from build123d import *

# Parameters (mm, degrees)
SKETCH1_W           = 16.5
SKETCH1_H           = 16.5
BOSS_EXTRUDE2_DEPTH = 7.5
SKETCH2_W           = 16.5
SKETCH2_H           = 10.25
CUT_EXTRUDE1_DEPTH  = 33.450924486
SKETCH5_W           = 4
SKETCH5_H           = 37
BOSS_EXTRUDE4_DEPTH = 7.5
SKETCH4_R           = 1.75
BOSS_EXTRUDE3_DEPTH = 2
FILLET1_R           = 3
FILLET2_R           = 1
FILLET3_R           = 1


with BuildPart() as part:
    # Sketch1 → Boss-Extrude2 (new body)
    with BuildSketch(Plane(origin=(0, 0, 0), x_dir=(1, 0, 0), z_dir=(0, 1, 0))):
        Polygon((-11.25, -11.25), (-11.25, 11.25), (-9.05, 29.5), (-6.05, 29.5), (-6.05, 24.5), (6.05, 24.5), (6.05, 29.5), (9.05, 29.5), (11.25, 11.25), (11.25, -11.25), (9.05, -29.5), (6.05, -29.5), (6.05, -24.5), (-6.05, -24.5), (-6.05, -29.5), (-9.05, -29.5), align=None)
        Rectangle(SKETCH1_W, SKETCH1_H, mode=Mode.SUBTRACT)
    extrude(amount=BOSS_EXTRUDE2_DEPTH)

    # Sketch2 → Cut-Extrude1 (cut, through all)
    with BuildSketch(Plane(origin=(0, 7.5, 0), x_dir=(1, 0, 0), z_dir=(0, 1, 0))):
        with Locations((0, 13.375)):
            Rectangle(SKETCH2_W, SKETCH2_H)
        with Locations((0, -13.375)):
            Rectangle(SKETCH2_W, SKETCH2_H)
    extrude(amount=-CUT_EXTRUDE1_DEPTH, mode=Mode.SUBTRACT)

    # Sketch5 → Boss-Extrude4 (add)
    with BuildSketch(Plane(origin=(0, 7.5, 0), x_dir=(1, 0, 0), z_dir=(0, 1, 0))):
        Rectangle(SKETCH5_W, SKETCH5_H)
    extrude(amount=-BOSS_EXTRUDE4_DEPTH)

    # Sketch4 → Boss-Extrude3 (add)
    with BuildSketch(Plane.XY.offset(24.5)):
        with BuildLine():
            Line((-3.8, 7.5), (3.7, 7.5))
            Line((3.7, 7.5), (3.7, 15))
            ThreePointArc((3.7, 15), (-0.05, 18.75), (-3.8, 15))
            Line((-3.8, 15), (-3.8, 7.5))
        make_face()
        with Locations((-0.05, 15)):
            Circle(SKETCH4_R, mode=Mode.SUBTRACT)
    boss_extrude3 = extrude(amount=-BOSS_EXTRUDE3_DEPTH)

    # Mirror1: Boss-Extrude3 across plane
    add(boss_extrude3.mirror(Plane.XY))

    # Fillet1
    fillet1_edges = [part.edges().sort_by_distance(p)[0] for p in [
        (-8.25, 3.75, -18.5),
        (8.25, 3.75, -18.5),
        (8.25, 3.75, 18.5),
        (-8.25, 3.75, 18.5),
    ]]
    fillet(fillet1_edges, radius=FILLET1_R)

    # Fillet2
    fillet2_edges = [part.edges().sort_by_distance(p)[0] for p in [
        (-3.8, 7.5, 23.5),
        (3.7, 7.5, 23.5),
        (-3.8, 7.5, -23.5),
        (3.7, 7.5, -23.5),
    ]]
    fillet(fillet2_edges, radius=FILLET2_R)

    # Fillet3
    fillet3_edges = [part.edges().sort_by_distance(p)[0] for p in [
        (-2, 7.5, 0),
        (2, 7.5, 0),
        (-2, 0, 0),
        (2, 0, 0),
    ]]
    fillet(fillet3_edges, radius=FILLET3_R)


solid = part.part
Read the model definition and answer for the solid it produces. Units are mm, in the model's axes. A direction names the side the tool comes from. Round coordinates to 2 decimals unless told otherwise and drop trailing zeros. Order: outer loops, then holes, each group sorted by start corner. A loop starts at its lowest first (then second) coordinate and runs counter-clockwise, first axis right, second up.
1) The part is cut by section A-A on y = 9.5. Write down the section's boundary in (x, z), plus the area to 3 significant figures.
2) The part is cut by section D-D on y = 3.75. Write down the section's boundary in (x, z), plus the area to 3 significant figures.
3) For faces 1 (the face through (8.25, 4, 0)), 2 (the face through (3.7, 12, -24)), 3 (the face through (6.05, 4, -27)), determine the directions among +Z, -Z, +X, -X, +Y, -Y from which every point of the face is accessible in a straight line to the end or side of a thin tool.
4) The part is cut by section C-C on z = -26. Write down the section's boundary in (x, y), plus the area to 3 significant figures.
5) Flat-ended cylindrical pins translate along their axes: pin 1 (8 mm diameter, centred on x = 4.5, z = -2.5, fed in from -Y); pin 2 (2.5 mm diameter, centred on y = 5, z = -26, fed in from +X); pin 3 (4 mm diameter, centred on x = 5.5, y = 12.5, fed in from -Z); pin 4 (4 mm diameter, centred on y = 3, z = 26, fed in from -X). Find the tip coordinate at first contact, or state that the pin passes through.
6) Straight lines are drawn through the part: L1, parallel to X at y = 4, z = -2; L2, parallel to Y at x = -0.05, z = -22.9; L3, parallel to Z at x = -3, y = 12.5. For each, find the intervals that lie inside material, in ascending order.
7) The part is cut by section B-B on x = -0.05. Write down the section's boundary in (y, z).
8) The mould has two halves that part along X. Classify faces 4 (the face through (3.7, 12, 24)), 5 (the face through (0, 7, -24.5)), 6 (the face through (-8, 4, -29.5)): released by +X, released by -X, zero draft, split by the parting line, or undercut.
Resolved:
1. outline: (-3.8, -24.5) - (3.7, -24.5) - (3.7, -22.5) - (-3.8, -22.5) - close; (-3.8, 22.5) - (3.7, 22.5) - (3.7, 24.5) - (-3.8, 24.5) - close
1. area: 30.0 mm2
2. outline: (-11.25, -11.25) - (-9.05, -29.5) - (-6.05, -29.5) - (-6.05, -24.5) - (6.05, -24.5) - (6.05, -29.5) - (9.05, -29.5) - (11.25, -11.25) - (11.25, 11.25) - (9.05, 29.5) - (6.05, 29.5) - (6.05, 24.5) - (-6.05, 24.5) - (-6.05, 29.5) - (-9.05, 29.5) - (-11.25, 11.25) - close; hole (-8.25, -15.5) arc R3 ccw to (-5.25, -18.5) - (-2, -18.5) - (-2, 18.5) - (-5.25, 18.5) arc R3 ccw to (-8.25, 15.5) - close; hole (2, -18.5) - (5.25, -18.5) arc R3 ccw to (8.25, -15.5) - (8.25, 15.5) arc R3 ccw to (5.25, 18.5) - (2, 18.5) - close
2. area: 671 mm2
3. face 1: +Y, -Y
3. face 2: +Z, -Z, +X, +Y
3. face 3: -Z, +Y, -Y
4. outline: (-9.47, 0) - (-6.05, 0) - (-6.05, 7.5) - (-9.47, 7.5) - close; (6.05, 0) - (9.47, 0) - (9.47, 7.5) - (6.05, 7.5) - close
4. area: 51.3 mm2
5. pin 1: stops at y = 0
5. pin 2: stops at x = 9.62
5. pin 3: stops at z = -24.5
5. pin 4: stops at x = -9.71
6. L1: x = -11.25 to -8.25, -2 to 2, 8.25 to 11.25
6. L2: y = 0 to 13.25, 16.75 to 18.75
6. L3: z = -24.5 to -22.5, 22.5 to 24.5
7. outline: (0, -24.5) - (13.25, -24.5) - (13.25, -22.5) - (7.5, -22.5) - (7.5, 22.5) - (13.25, 22.5) - (13.25, 24.5) - (0, 24.5) - close; (16.75, -24.5) - (18.75, -24.5) - (18.75, -22.5) - (16.75, -22.5) - close; (16.75, 22.5) - (18.75, 22.5) - (18.75, 24.5) - (16.75, 24.5) - close
8. face 4: released by +X
8. face 5: undercut
8. face 6: zero draft
